Check sheet for the drawn part. Datum: minimum x, y, z corner. Units: mm. Coordinates: 2 decimals unless noted, no trailing zeros. Write each loop counter-clockwise with the first axis right and the second up, starting at its lowest first coordinate (ties: lowest second). Pieces come first, ordered by that corner, then holes. Notation, with made-up numbers: (18.25, 28) - (32.25, 28) arc R28 cw to (32.25, 67) - close; hole circle Ø6 at (87, 4). An arc over 180 degrees is marked (long way). Use one line per item in the form item = value. Start each with the question number.
1. Cross-section at C-C on x = 17. Record the boundary of the cut face in (y, z) (3 decimals).
2. Draft check along Z on the marked faces 1, 2, 3 and 4. Enter one of: +Z half, -Z half, draft (parallel to the pull), parting line (faces both ways), or undercut.
3. Cross-section at A-A on x = 75. Record the boundary of the cut face in (y, z) (3 decimals).
4. Scan lines: line 1 along Y through (x, z) = (17, 2.4) (3 decimals); line 2 along Z through (x, y) = (75, 3.75) (3 decimals); line 3 along X through (y, z) = (2.25, 2.75) (1 decimal). Record each from-to range of solid material in increasing order.
5. Cross-section at B-B on z = 12.5. Record the boundary of the cut face in (x, y).
6. Cross-section at D-D on y = 4. Record the boundary of the cut face in (x, z) (3 decimals), then the cut area to 3 significant figures.
7. Go/stop test with flat-tipped pins: pin 1 Ø5.5 at (x, z) = (75, 9.525) entering from +Y; pin 2 Ø1.6 at (x, y) = (67.5, 3) entering from -Z. Record where each tip stops, or that it passes through.
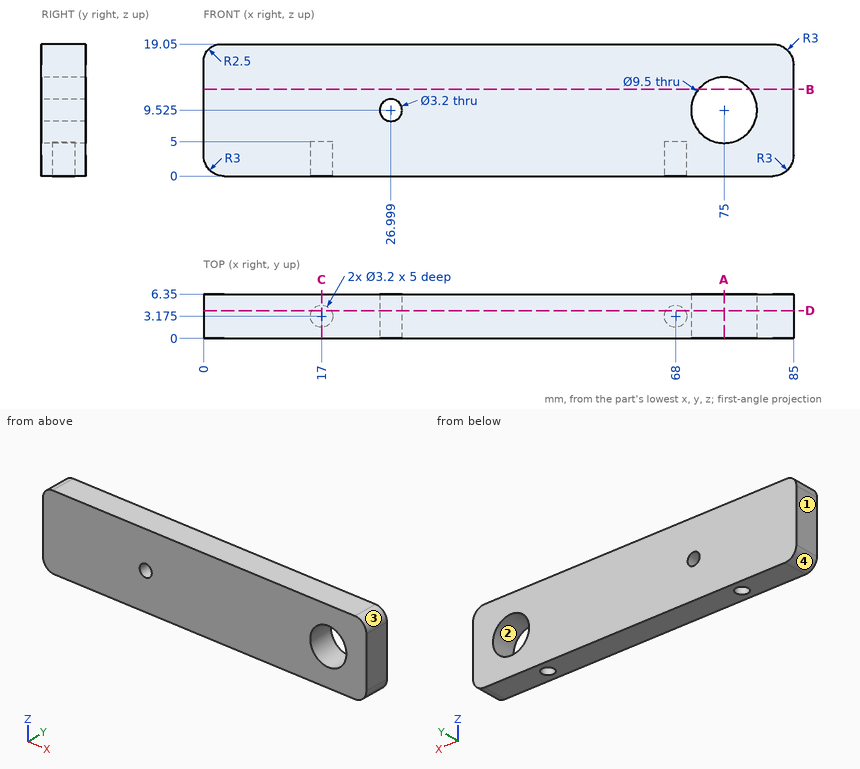
Final values:
q1.outline = (0, 0) - (1.575, 0) - (1.575, 5) - (4.775, 5) - (4.775, 0) - (6.35, 0) - (6.35, 19.05) - (0, 19.05) - close
q2.face_1 = draft
q2.face_2 = undercut
q2.face_3 = +Z half
q2.face_4 = -Z half
q3.outline = (0, 0) - (6.35, 0) - (6.35, 4.775) - (0, 4.775) - close; (0, 14.275) - (6.35, 14.275) - (6.35, 19.05) - (0, 19.05) - close
q4.line_1 = 0 to 1.575, 4.775 to 6.35
q4.line_2 = 0 to 4.775, 14.275 to 19.05
q4.line_3 = 0 to 15.7, 18.3 to 66.7, 69.3 to 85
q5.outline = (0, 0) - (71.3, 0) - (71.3, 6.35) - (0, 6.35) - close; (78.7, 0) - (85, 0) - (85, 6.35) - (78.7, 6.35) - close
q6.outline = (0, 3) arc R3 ccw to (3, 0) - (15.629, 0) - (15.629, 5) - (18.371, 5) - (18.371, 0) - (66.629, 0) - (66.629, 5) - (69.371, 5) - (69.371, 0) - (82, 0) arc R3 ccw to (85, 3) - (85, 16.05) arc R3 ccw to (82, 19.05) - (2.5, 19.05) arc R2.5 ccw to (0, 16.55) - close; hole circle Ø3.2 at (26.999, 9.525); hole circle Ø9.5 at (75, 9.525)
q6.area = 1,510 mm²
q7.pin_1 = through
q7.pin_2 = 5
